Read the model definition and answer for the solid it produces. Units are mm, in the model's axes. Face numbers are marked on the shaded views. A direction names the side the tool comes from. Round coordinates to 2 decimals unless told otherwise and drop trailing zeros. Write each loop counter-clockwise with the first axis right and the second up, starting at its lowest first coordinate (ties: lowest second). Pieces come first, ordered by that corner, then holes. Notation, with made-up numbers: (-12.5, 57) - (21.5, 57) arc R20 ccw to (21.5, 74) - close; hole circle Ø3 at (38.5, 6). An arc over 180 degrees is marked (long way). Answer as CSV lines item,"result". Start each with the question number.
1) Which of the six approach directions +Z, -Z, +X, -X, +Y, -Y give full straight-line access (tool end or side, diameter ignored) to the marked faces 1 and 2?
2) Find section A-A on x = -30. Determine the outline of the cut face in (y, z).
3) Each of these flat-tipped pins is pushed along its axis until it touches: pin 1 (3 mm diameter, centred on x = -3, z = -4.5, fed in from -Y); pin 2 (2 mm diameter, centred on x = -50, z = -3, fed in from +Y). Where does it stop, or does it pass through?
4) Find section C-C on y = 14.5. Determine the outline of the cut face in (x, z).
5) Consider line 1 along Y through (x, z) = (-15, -2); line 2 along X through (y, z) = (34, -3); line 3 along Z through (x, y) = (-10, 34.25). Determine where each line is inside the solid, lowest interval first.
6) Find section D-D on y = 37.5. Determine the outline of the cut face in (x, z), then the cut area to 3 significant figures.
7) Find section B-B on z = -5.35. Determine the outline of the cut face in (x, y), then the cut area to 3 significant figures.
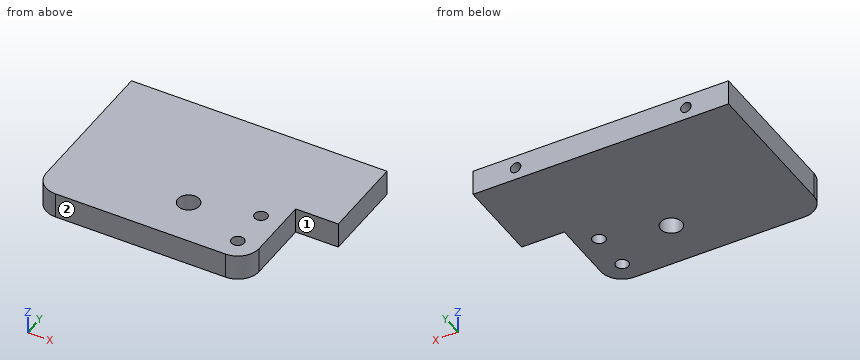
Autodesk Inventor part; units mm, degrees
ref_plane "YZ Plane" through (0, 0, 0) normal (1, 0, 0) x (0, 1, 0)
ref_plane "XZ Plane" through (0, 0, 0) normal (0, 1, 0) x (-1, 0, 0)
ref_plane "XY Plane" through (0, 0, 0) normal (0, 0, 1) x (1, 0, 0)
sketch "Sketch1" plane through (0, 0, 0) normal (0, 1, 0) x (-1, 0, 0)
  line L0 (0, 0) -> (60, 0)
  line L1 (60, 0) -> (60, -6)
  line L2 (60, -6) -> (0, -6)
  line L3 (0, -6) -> (0, 0)
  dimension "d7" = 60
  dimension "d8" = 6
extrude "Extrusion1" add sketch "Sketch1" along normal blind 40
sketch "Sketch2" plane through (0, 0, -6) normal (0, 0, -1) x (-1, 0, 0)
  circle A0 centre (30, 11) radius 2.5
  line L0 (0, 40) -> (60, 40)
  line L1 (0, 0) -> (0, 40)
  line L2 (0, 0) -> (60, 0)
  dimension "d2" = 5
  dimension "d3" = 29
  dimension "d4" = 30
extrude "Extrusion2" cut sketch "Sketch2" against normal blind 10
fillet "Fillet1" radius 5 2 edges at (-60, 0, -3) (0, 0, -3)
sketch "Sketch3" plane through (-60, 40, 0) normal (0, 0, 1) x (1, 0, 0)
  circle A0 centre (45, -35) radius 1.5
  circle A1 centre (45, -25.5) radius 1.5
  line L0 (5, -40) -> (55, -40)
  line L1 (60, -35) -> (60, 0)
  point P0 (60, -40)
  dimension "d16" = 5
  dimension "d17" = 9.5
  dimension "d18" = 15
  dimension "d20" = 3
  dimension "d21" = 3
  dimension "d42" = 15
hole "Hole1" at (-15, 5, 0) at (-15, 14.5, 0) direction (0, 0, -1) diameter 3 end through all
sketch "Sketch4" plane through (0, 40, 0) normal (0, 1, 0) x (1, 0, 0)
  circle A0 centre (-10, 2.5) radius 1.5
  circle A1 centre (-50, 2.5) radius 1.5
  circle A2 centre (-50, 3) radius 1.5
  circle A3 centre (-10, 3) radius 1.5
  line L0 (-60, 0) -> (0, 0)
  line L1 (-60, 6) -> (-60, 0)
  line L2 (0, 0) -> (0, 6)
  dimension "d36" = 3
  dimension "d37" = 3
  dimension "d38" = 10
  dimension "d39" = 10
  dimension "d40" = 3
  dimension "d41" = 3
hole "Hole2" at (-50, 40, -3) at (-10, 40, -3) direction (0, -1, 0) diameter 2.459 depth 8.8 tip angle 118
sketch "Sketch5" plane through (-60, 40, 0) normal (0, 0, 1) x (1, 0, 0)
  line L0 (70, -50) -> (50, -50)
  line L1 (50, -50) -> (50, -20)
  line L2 (50, -20) -> (70, -20)
  line L3 (70, -20) -> (70, -50)
  line L4 (5, -40) -> (55, -40)
  line L5 (60, -35) -> (60, 0)
  point P0 (60, -40)
  dimension "d43" = 10
  dimension "d44" = 10
  dimension "d45" = 20
  dimension "d46" = 10
extrude "Extrusion3" cut sketch "Sketch5" against normal blind 10
fillet "Fillet2" radius 5 1 edges at (-10, 0, -3)
equation "\"d22\" = d20"
properties part number "X-Axis_beltplates"
Check values:
1,face 1,"+Z, -Z, +X, -Y"
1,face 2,"+Z, -Z, +X, -X, -Y"
2,outline,"(0, -6) - (8.5, -6) - (8.5, 0) - (0, 0) - close; (13.5, -6) - (40, -6) - (40, 0) - (13.5, 0) - close"
3,pin 1,"stops at y = 20"
3,pin 2,"stops at y = 31.06"
4,outline,"(-60, -6) - (-16.5, -6) - (-16.5, 0) - (-60, 0) - close; (-13.5, -6) - (-10, -6) - (-10, 0) - (-13.5, 0) - close"
5,line 1,"y = 0 to 3.5, 6.5 to 13, 16 to 40"
5,line 2,"x = -60 to -51.23, -48.77 to -11.23, -8.77 to 0"
5,line 3,"z = -6 to -4.23, -1.77 to 0"
6,outline,"(-60, -6) - (0, -6) - (0, 0) - (-60, 0) - close; hole circle Ø2.46 at (-50, -3); hole circle Ø2.46 at (-10, -3)"
6,area,"351 mm^2"
7,outline,"(-60, 5) arc R5 ccw to (-55, 0) - (-15, 0) arc R5 ccw to (-10, 5) - (-10, 20) - (0, 20) - (0, 40) - (-60, 40) - close; hole circle Ø5 at (-30, 11); hole circle Ø3 at (-15, 5); hole circle Ø3 at (-15, 14.5)"
7,area,"2,160 mm^2"
